Geometry check sheet. Reference: the model listing, model coordinates, mm. A direction names the side the tool comes from. Give positions to 0.01 mm unless a question says otherwise; leave off trailing zeros. Loops run counter-clockwise (first coordinate to the right, second up) from the corner with the lowest first, then second, coordinate; pieces in that order, holes last. Notation, with made-up numbers: (76, -20) -> (127, -20) arc R12 ccw to (127, -15) -> close; hole circle Ø10 at (67, 67). An arc over 180 degrees is marked (long way). Write item = value, one per line.
```python
from build123d import *

# Parameters (mm, degrees)
SKETCH1_W               = 65.26
SKETCH1_H               = 75
BOSS_EXTRUDE1_DEPTH     = 43
CUT_EXTRUDE1_DEPTH      = 35
CUT_EXTRUDE1_DEPTH_BACK = 35
SKETCH4_W               = 7
SKETCH4_H               = 1.7
CUT_EXTRUDE2_DEPTH      = 41.5
SKETCH5_W               = 7
SKETCH5_H               = 14
SKETCH5_H_2             = 15
SKETCH5_W_2             = 4.5
SKETCH5_H_3             = 9
CUT_EXTRUDE3_DEPTH      = 65.755053085
SKETCH7_W               = 6
SKETCH7_H               = 12
CUT_EXTRUDE4_DEPTH      = 92.75705368
FILLET1_R               = 1
BOSS_EXTRUDE2_DEPTH     = 10
CUT_EXTRUDE5_DEPTH      = 20
CUT_EXTRUDE5_DEPTH_BACK = 20
SKETCH12_W              = 72.6
SKETCH12_H              = 2
CUT_EXTRUDE6_DEPTH      = 64
SKETCH13_W              = 6.500006658
SKETCH13_H              = 70
CUT_EXTRUDE7_DEPTH      = 3
BOSS_EXTRUDE3_DEPTH     = 7
SKETCH17_R              = 2
CUT_EXTRUDE9_DEPTH      = 2.5


with BuildPart() as part:
    # Sketch1 → Boss-Extrude1 (new body)
    with BuildSketch(Plane(origin=(0, 0, 0), x_dir=(1, 0, 0), z_dir=(0, 1, 0))):
        Rectangle(SKETCH1_W, SKETCH1_H)
    extrude(amount=BOSS_EXTRUDE1_DEPTH)

    # Sketch3 → Cut-Extrude1 (cut, two sides: drawn at the far end of the back side and taken through both)
    with BuildSketch(Plane.XY.offset(-CUT_EXTRUDE1_DEPTH_BACK)):
        with BuildLine():
            Line((30.629993342, 0), (-30.63, 0))
            Line((-30.63, 0), (-30.63, 31.95))
            ThreePointArc((-30.63, 31.95), (-24.219797365, 40.606440947), (-14.070006658, 37))
            Line((-14.070006658, 37), (-10.739993342, 37))
            ThreePointArc((-10.739993342, 37), (-3.23, 41), (4.279993342, 37))
            Line((4.279993342, 37), (7.610006658, 37))
            ThreePointArc((7.610006658, 37), (15.12, 41), (22.629993342, 37))
            Line((22.629993342, 37), (23.629993342, 37))
            Line((23.629993342, 37), (23.629993342, 41.5))
            Line((23.629993342, 41.5), (30.629993342, 41.5))
            Line((30.629993342, 41.5), (30.629993342, 0))
        make_face()
    extrude(amount=CUT_EXTRUDE1_DEPTH + CUT_EXTRUDE1_DEPTH_BACK, mode=Mode.SUBTRACT)

    # Sketch4 → Cut-Extrude2 (cut)
    with BuildSketch(Plane(origin=(0, 0, 0), x_dir=(-1, 0, 0), z_dir=(0, -1, 0))):
        with Locations((-27.129993342, 35.85)):
            Rectangle(SKETCH4_W, SKETCH4_H)
    extrude(amount=-CUT_EXTRUDE2_DEPTH, mode=Mode.SUBTRACT)

    # Sketch5 → Cut-Extrude3 (cut, through all)
    with BuildSketch(Plane(origin=(0, 41.5, 0), x_dir=(-1, 0, 0), z_dir=(0, -1, 0))):
        with Locations((-27.129993342, -13.3)):
            Rectangle(SKETCH5_W, SKETCH5_H)
        with Locations((-27.129993342, 22.2)):
            Rectangle(SKETCH5_W, SKETCH5_H_2)
        with Locations((-26.879993342, 4.2)):
            Rectangle(SKETCH5_W_2, SKETCH5_H_3)
    extrude(amount=-CUT_EXTRUDE3_DEPTH, mode=Mode.SUBTRACT)

    # Sketch7 → Cut-Extrude4 (cut, through all)
    with BuildSketch(Plane.XY.offset(-36.7)):
        with BuildLine():
            Line((23.629993342, 29.5), (30.629993342, 29.5))
            Line((30.629993342, 29.5), (30.629993342, 32))
            Line((30.629993342, 32), (29.323734439, 32))
            ThreePointArc((29.323734439, 32), (27.129993342, 30.25), (24.936252245, 32))
            Line((24.936252245, 32), (23.629993342, 32))
            Line((23.629993342, 32), (23.629993342, 29.5))
        make_face()
        with BuildLine():
            Line((23.629993342, 35.5), (30.629993342, 35.5))
            Line((30.629993342, 35.5), (30.629993342, 33))
            Line((30.629993342, 33), (29.323734439, 33))
            ThreePointArc((29.323734439, 33), (27.129993342, 34.75), (24.936252245, 33))
            Line((24.936252245, 33), (23.629993342, 33))
            Line((23.629993342, 33), (23.629993342, 35.5))
        make_face()
        with Locations((27.629993342, 20.5)):
            Rectangle(SKETCH7_W, SKETCH7_H)
    extrude(amount=-CUT_EXTRUDE4_DEPTH, mode=Mode.SUBTRACT)

    # Fillet1
    fillet1_edges = [part.edges().sort_by_distance(p)[0] for p in [
        (0, 43, -37.5),
        (32.63, 43, 0),
        (0, 43, 37.5),
        (-32.63, 43, 0),
        (29.129993342, 43, -4.2),
        (26.879993342, 43, -8.7),
        (24.629993342, 43, -4.2),
        (26.879993342, 43, 0.3),
        (30.629993342, 43, -22.2),
        (27.129993342, 43, -29.7),
        (23.629993342, 43, -22.2),
        (27.129993342, 43, -14.7),
        (30.629993342, 43, 13.3),
        (27.129993342, 43, 6.3),
        (23.629993342, 43, 13.3),
        (27.129993342, 43, 20.3),
        (32.63, 21.5, 37.5),
        (32.63, 21.5, -37.5),
        (-32.63, 21.5, 37.5),
        (-32.63, 21.5, -37.5),
    ]]
    fillet(fillet1_edges, radius=FILLET1_R - 0.0001)  # a hair under: the kernel refuses the full size

    # Sketch8 → Boss-Extrude2 (add)
    with BuildSketch(Plane(origin=(0, 0, 0), x_dir=(-1, 0, 0), z_dir=(0, -1, 0))):
        with BuildLine():
            Line((-30.629993342, 7), (-29.129993342, 7))
            ThreePointArc((-29.129993342, 7), (-26.129993342, 10), (-29.129993342, 13))
            Line((-29.129993342, 13), (-30.629993342, 13))
            Line((-30.629993342, 13), (-30.629993342, 7))
        make_face()
        with BuildLine():
            Line((-30.629993342, -13), (-29.129993342, -13))
            ThreePointArc((-29.129993342, -13), (-26.129993342, -10), (-29.129993342, -7))
            Line((-29.129993342, -7), (-30.629993342, -7))
            Line((-30.629993342, -7), (-30.629993342, -13))
        make_face()
    extrude(amount=-BOSS_EXTRUDE2_DEPTH)

    # Sketch11 → Cut-Extrude5 (cut, two sides: drawn at the far end of the back side and taken through both)
    with BuildSketch(Plane.XY.offset(-CUT_EXTRUDE5_DEPTH_BACK)):
        Polygon((30.629993342, 10), (26.129993342, 6), (26.129993342, 10), align=None)
    extrude(amount=CUT_EXTRUDE5_DEPTH + CUT_EXTRUDE5_DEPTH_BACK, mode=Mode.SUBTRACT)

    # Sketch12 → Cut-Extrude6 (cut)
    with BuildSketch(Plane(origin=(32.63, 0, 0), x_dir=(0, 0, -1), z_dir=(1, 0, 0))):
        with Locations((0, 2)):
            Rectangle(SKETCH12_W, SKETCH12_H)
    extrude(amount=-CUT_EXTRUDE6_DEPTH, mode=Mode.SUBTRACT)

    # Sketch13 → Cut-Extrude7 (cut)
    with BuildSketch(Plane.XZ):
        with Locations((29.379996671, 0)):
            Rectangle(SKETCH13_W, SKETCH13_H)
    extrude(amount=-CUT_EXTRUDE7_DEPTH, mode=Mode.SUBTRACT)

    # Sketch15 → Boss-Extrude3 (add)
    with BuildSketch(Plane(origin=(23.629993342, 0, 0), x_dir=(0, 0, -1), z_dir=(1, 0, 0))):
        Polygon((36.7, 0), (36.7, 3), (36.3, 3), (36.3, 1), (35, 1), (35, 0), align=None)
    extrude(amount=BOSS_EXTRUDE3_DEPTH)

    # Sketch17 → Cut-Extrude9 (cut)
    with BuildSketch(Plane(origin=(0, 3, 0), x_dir=(-1, 0, 0), z_dir=(0, -1, 0))):
        with Locations(Location((-29.129993342, 10, 0), (0, 0, 90))):
            Circle(SKETCH17_R)
        with Locations(Location((-29.129993342, -10, 0), (0, 0, 90))):
            Circle(SKETCH17_R)
    extrude(amount=-CUT_EXTRUDE9_DEPTH, mode=Mode.SUBTRACT)


solid = part.part
```
Item 1: Draft check along Y on faces 4 (the cylindrical face through (27.178, 4.232, 10.434)), 5 (the cylindrical face through (27.17, 30.25, -37.09)), 6 (the flat face through (6, 37, 0)). Enter one of: +Y half, -Y half, draft (parallel to the pull), parting line (faces both ways), or undercut.
Answer:
face_4 = draft
face_5 = undercut
face_6 = -Y half
Item 2: Section check D-D, the plane z = 27.5. Record the cut outline in (x, y), plus the area to 3 significant figures.
Answer:
outline = (-32.63, 0) -> (-30.63, 0) -> (-30.63, 1) -> (-31.37, 1) -> (-31.37, 3) -> (-30.63, 3) -> (-30.63, 31.95) arc R9.05 cw to (-14.07, 37) -> (-10.74, 37) arc R9.05 cw to (4.28, 37) -> (7.61, 37) arc R9.05 cw to (22.63, 37) -> (23.63, 37) -> (23.63, 41.5) -> (30.63, 41.5) -> (30.63, 3) -> (32.63, 3) -> (32.63, 42) arc R1 ccw to (31.63, 43) -> (-31.63, 43) arc R1 ccw to (-32.63, 42) -> close
area = 376 mm^2
Item 3: Gauge pin test, flat ends, axial feed: pin 1 (1.5 mm diameter, centred on x = 17, z = 2, fed in from -Y); pin 2 (1.1 mm diameter, centred on y = 0.5, z = -13, fed in from +X); pin 3 (0.6 mm diameter, centred on y = 19.5, z = -37, fed in from +X). Record the tip position at first contact, or that the pin passes through.
Answer:
pin_1 = 40.61
pin_2 = -30.63
pin_3 = 32.61
Item 4: Section check C-C, the plane x = -13. Record the cut outline in (y, z), plus the area to 3 significant figures.
Answer:
outline = (0, -37.5) -> (42, -37.5) arc R1 ccw to (43, -36.5) -> (43, 36.5) arc R1 ccw to (42, 37.5) -> (0, 37.5) -> (0, 35) -> (1, 35) -> (1, 36.3) -> (3, 36.3) -> (3, 35) -> (37, 35) -> (37, -35) -> (3, -35) -> (3, -36.3) -> (1, -36.3) -> (1, -35) -> (0, -35) -> close
area = 629 mm^2
Item 5: Section check B-B, the plane y = 4.5. Record the cut outline in (x, z).
Answer:
outline = (-32.63, -36.5) arc R1 ccw to (-31.63, -37.5) -> (31.63, -37.5) arc R1 ccw to (32.63, -36.5) -> (32.63, 36.5) arc R1 ccw to (31.63, 37.5) -> (-31.63, 37.5) arc R1 ccw to (-32.63, 36.5) -> close; hole (-30.63, -35) -> (23.63, -35) -> (23.63, -36.7) -> (30.63, -36.7) -> (30.63, -13) -> (29.13, -13) arc R3 cw to (29.13, -7) -> (30.63, -7) -> (30.63, 7) -> (29.13, 7) arc R3 cw to (29.13, 13) -> (30.63, 13) -> (30.63, 35) -> (-30.63, 35) -> close; hole circle Ø4 at (29.13, -10); hole circle Ø4 at (29.13, 10)
Item 6: Tool access check on faces 1 (the flat face through (27, 38, -36.7)), 2 (the cylindrical face through (27.178, 4.232, -9.566)), 3 (the flat face through (28.91, 8.47, 9.96)). Record the directions out of +Z, -Z, +X, -X, +Y, -Y that give a thin tool (end or side, any length) a straight path to the whole face; none if there is none.
Answer:
face_1 = none
face_2 = -Y
face_3 = +Y
Item 7: Thickness scan on L1, parallel to X at y = 4, z = -10; L2, parallel to Z at x = 8, y = 17; L3, parallel to X at y = 6, z = -17. Record the ranges inside material, lowest first. Write a range as [from, to].
Answer:
L1 = [-32.63, -30.63], [26.13, 27.13], [31.13, 32.63]
L2 = [-37.5, -35], [35, 37.5]
L3 = [-32.63, -30.63], [30.63, 32.63]
